```python
from build123d import *

# Parameters (mm, degrees)
BOSS_EXTRU_1_DEPTH      = 18
BOSS_EXTRU_1_DEPTH_BACK = 18
CONG_1_R                = 10


with BuildPart() as part:
    # Esquisse1 → Boss.-Extru.1 (new body, two sides)
    with BuildSketch(Plane.XY) as boss_extru_1_sk:
        Polygon((0, 0), (0, 80), (13.680805733, 117.587704831), (16.499883595, 116.561644401), (3.192533317, 80), (3.192533317, 0), align=None)
    extrude(amount=BOSS_EXTRU_1_DEPTH)
    extrude(boss_extru_1_sk.sketch, amount=-BOSS_EXTRU_1_DEPTH_BACK)

    # Cong_1
    cong_1_edges = [part.edges().sort_by_distance(p)[0] for p in [
        (0, 80, 0),
    ]]
    fillet(cong_1_edges, radius=CONG_1_R)


solid = part.part
```
Input: part model. Units: mm. Frame: model coordinates. A direction names the side the tool comes from. Round coordinates to 2 decimals unless told otherwise and drop trailing zeros. Loops run counter-clockwise (first coordinate to the right, second up) from the corner with the lowest first, then second, coordinate; pieces in that order, holes last. Notation, with made-up numbers: (72.25, 11) -> (78.25, 11) arc R22 ccw to (78.25, 22) -> close; hole circle Ø8 at (13, 79). An arc over 180 degrees is marked (long way). One line per item, written item: value.
(1) Set-up query: faces 1 (the face through (3.193, 41, 0)), 2 (the face through (7.05, 99.37, 0.25)). Return all of +Z, -Z, +X, -X, +Y, -Y with unobstructed straight access to the full face (end or side cutting, diameter ignored); none if empty.
Geometry check:
face 1: +Z, -Z, +X, -Y
face 2: +Z, -Z, -X, +Y
(2) Pin query (flat end, axial travel): pin 1 (8 mm diameter, centred on y = 103, z = 13.5, fed in from -X); pin 2 (11 mm diameter, centred on y = 45.5, z = 8.5, fed in from +X); pin 3 (5 mm diameter, centred on y = 40, z = 12, fed in from -X); pin 4 (4 mm diameter, centred on x = 7, y = 49.5, fed in from -Z). Return the tip coordinate at first contact, or that it passes through.
Geometry check:
pin 1: x = 6.92
pin 2: x = 3.19
pin 3: x = 0
pin 4: through
(3) Section B-B (x = 6.5). Return the cut outline in (y, z), plus the area to 3 significant figures.
Geometry check:
outline: (89.09, -18) -> (97.86, -18) -> (97.86, 18) -> (89.09, 18) -> close
area: 316 mm2
(4) Section C-C (y = 93.5). Return the cut outline in (x, z), plus the area to 3 significant figures.
Geometry check:
outline: (4.91, -18) -> (8.11, -18) -> (8.11, 18) -> (4.91, 18) -> close
area: 115 mm2
(5) Material intervals for line 1 (X direction, y = 15, z = 10); line 2 (X direction, y = 92, z = 5), sorted ascending. Write a range as [from, to].
Geometry check:
line 1: [0, 3.19]
line 2: [4.37, 7.56]
(6) Section A-A (z = 12). Return the cut outline in (x, y).
Geometry check:
outline: (0, 0) -> (3.19, 0) -> (3.19, 80) -> (16.5, 116.56) -> (13.68, 117.59) -> (0.6, 81.66) arc R10 ccw to (0, 78.24) -> close
